from build123d import *

# Parameters (mm, degrees)
BOSS_EXTRUDE1_DEPTH = 2.5
BOSS_EXTRUDE2_DEPTH = 50.5


with BuildPart() as part:
    # Sketch1 → Boss-Extrude1 (new body)
    with BuildSketch(Plane.XY):
        Polygon((-50.5, 9.5), (-50.5, -7), (-40.5, -7), (-39, -5.5), (-37.5, -7), (-27.5, -7), (-26, -5.5), (-24.5, -7), (-14.5, -7), (-13, -5.5), (-11.5, -7), (-1.5, -7), (0, -5.5), (1.5, -7), (11.5, -7), (13, -5.5), (14.5, -7), (24.5, -7), (26, -5.5), (27.5, -7), (37.5, -7), (39, -5.5), (40.5, -7), (50.5, -7), (50.5, 9.5), align=None)
        Polygon((-40.5, -7), (-50.5, -7), (-50.5, 9.5), (-53, 9.5), (-53, -9.5), (53, -9.5), (53, 9.5), (50.5, 9.5), (50.5, -7), (40.5, -7), (39, -5.5), (37.5, -7), (27.5, -7), (26, -5.5), (24.5, -7), (14.5, -7), (13, -5.5), (11.5, -7), (1.5, -7), (0, -5.5), (-1.5, -7), (-11.5, -7), (-13, -5.5), (-14.5, -7), (-24.5, -7), (-26, -5.5), (-27.5, -7), (-37.5, -7), (-39, -5.5), align=None)
    extrude(amount=-BOSS_EXTRUDE1_DEPTH)

    # Sketch1_3 → Boss-Extrude2 (add)
    with BuildSketch(Plane.XY):
        Polygon((-40.5, -7), (-50.5, -7), (-50.5, 9.5), (-53, 9.5), (-53, -9.5), (53, -9.5), (53, 9.5), (50.5, 9.5), (50.5, -7), (40.5, -7), (39, -5.5), (37.5, -7), (27.5, -7), (26, -5.5), (24.5, -7), (14.5, -7), (13, -5.5), (11.5, -7), (1.5, -7), (0, -5.5), (-1.5, -7), (-11.5, -7), (-13, -5.5), (-14.5, -7), (-24.5, -7), (-26, -5.5), (-27.5, -7), (-37.5, -7), (-39, -5.5), align=None)
    extrude(amount=BOSS_EXTRUDE2_DEPTH)

    # Mirror4: part across plane


with BuildPart() as part_1:
    add(part.part)
    add(part.part.mirror(Plane.XY.offset(50.5)))


solid = part_1.part
Design review of the part built by this model. Coordinates are the model's own, in mm. A direction names the side the tool comes from. Coordinates: 2 decimals unless noted, no trailing zeros. Order: outer loops, then holes, each group sorted by start corner. A loop starts at its lowest first (then second) coordinate and runs counter-clockwise, first axis right, second up.
Item 1: For faces 4 (the flat face through (4.2, 9.5, -0.3)), 5 (the flat face through (7, -7, 51)), list the 3-axis set-ups (+Z, -Z, +X, -X, +Y, -Y) from which the entire face can be reached by the end or side of a thin tool; tool diameter is ignored.
Item 2: Take a section at C-C, the plane x = -19. Write out the cut boundary in (y, z).
Item 3: For pin 1 Ø1.5 at (x, z) = (-10.5, 51.5) entering from +Y; pin 2 Ø8 at (x, z) = (18, 53.5) entering from +Y; pin 3 Ø8 at (x, z) = (23.5, 79.5) entering from +Y, all flat-tipped, find the tip position at first contact; note any pin that passes through.
Item 4: Take a section at A-A, the plane y = -3. Write out the cut boundary in (x, z), then the cut area to 4 significant figures.
Item 5: The part is to be moulded in two halves that separate along X. For faces 1 (the flat face through (-53, 0, 51)), 2 (the flat face through (-1, 0, -2.5)), 3 (the flat face through (-50.5, 1, 51)), say which applies: pulls with the +X half, pulls with the -X half, needs draft (parallel to the pull), parting line crosses it, or undercut.
Item 6: For line 1 (X direction, y = -2.25, z = 67); line 2 (Z direction, x = 48.5, y = 6.75); line 3 (Y direction, x = 37, z = 71), list the stretches that pass through material, from the lowest coordinate up.
The answers:
1. face 4: +Z, -Z, +X, -X, +Y
1. face 5: +Y
2. outline: (-9.5, -2.5) - (9.5, -2.5) - (9.5, 0) - (-7, 0) - (-7, 101) - (9.5, 101) - (9.5, 103.5) - (-9.5, 103.5) - close
3. pin 1: stops at y = -7
3. pin 2: stops at y = -6.5
3. pin 3: stops at y = -5.5
4. outline: (-53, -2.5) - (53, -2.5) - (53, 103.5) - (-53, 103.5) - close; hole (-50.5, 0) - (50.5, 0) - (50.5, 101) - (-50.5, 101) - close
4. area: 1,035 mm2
5. face 1: pulls with the -X half
5. face 2: needs draft
5. face 3: undercut
6. line 1: x = -53 to -50.5, 50.5 to 53
6. line 2: z = -2.5 to 0, 101 to 103.5
6. line 3: y = -9.5 to -7
